Design review of the part built by this model. Coordinates are the model's own, in mm. Coordinates: 2 decimals unless noted, no trailing zeros. Order: outer loops, then holes, each group sorted by start corner. A loop starts at its lowest first (then second) coordinate and runs counter-clockwise, first axis right, second up. Notation, with made-up numbers: M -29,-38 L -22,-38 A28 ccw -22,-2 Z; hole C 82,21 d2. An arc over 180 degrees is marked long. Answer in a Markdown table with one row per item.
from build123d import *

# Parameters (mm, degrees)
SKETCH1_W                         = 25.4
SKETCH1_H                         = 25.4
BOSS_EXTRUDE1_DEPTH               = 12.7
CHAMFER1_SIZE                     = 10.16
SKETCH2_R                         = 3.175
CUT_EXTRUDE1_DEPTH                = 25.4
SKETCH3_R                         = 3.175
CUT_EXTRUDE2_DEPTH                = 10.16
F_1_4_28_TAPPED_HOLE1_D           = 5.4102
F_1_4_28_TAPPED_HOLE1_DEPTH       = 15.494
F_1_4_28_TAPPED_HOLE1_CSINK_D     = 7.62
F_1_4_28_TAPPED_HOLE1_CSINK_ANGLE = 90
F_1_4_28_TAPPED_HOLE1_TIP         = 1.625388061


with BuildPart() as part:
    # Sketch1 → Boss-Extrude1 (new body)
    with BuildSketch(Plane.XY):
        with Locations((12.7, 12.7)):
            Rectangle(SKETCH1_W, SKETCH1_H)
    extrude(amount=BOSS_EXTRUDE1_DEPTH)

    # Chamfer1
    chamfer1_edges = [part.edges().sort_by_distance(p)[0] for p in [
        (0, 0, 6.35),
    ]]
    chamfer(chamfer1_edges, length=CHAMFER1_SIZE)

    # Sketch2 → Cut-Extrude1 (cut)
    with BuildSketch(Plane(origin=(0, 25.4, 0), x_dir=(1, 0, 0), z_dir=(0, 1, 0))):
        with Locations(Location((19.05, -6.35, 0), (0, 0, 270))):
            Circle(SKETCH2_R)
    extrude(amount=-CUT_EXTRUDE1_DEPTH, mode=Mode.SUBTRACT)

    # Sketch3 → Cut-Extrude2 (cut)
    with BuildSketch(Plane(origin=(5.08, 5.08, 0), x_dir=(0, 0, 1), z_dir=(-0.7071067811865488, -0.7071067811865462, 0))):
        with Locations(Location((6.35, 0, 0), (0, 0, 270))):
            Circle(SKETCH3_R)
    extrude(amount=-CUT_EXTRUDE2_DEPTH, mode=Mode.SUBTRACT)

    # 1/4-28 Tapped Hole1
    with Locations(Plane.XY.offset(12.7)):
        with Locations((8.980256121, 8.980256121), (18.974124868, 17.78)):
            CounterSinkHole(F_1_4_28_TAPPED_HOLE1_D / 2, F_1_4_28_TAPPED_HOLE1_CSINK_D / 2, depth=F_1_4_28_TAPPED_HOLE1_DEPTH, counter_sink_angle=F_1_4_28_TAPPED_HOLE1_CSINK_ANGLE)
            with Locations((0, 0, -(F_1_4_28_TAPPED_HOLE1_DEPTH + F_1_4_28_TAPPED_HOLE1_TIP / 2))):  # 118° drill point
                Cone(0, F_1_4_28_TAPPED_HOLE1_D / 2, F_1_4_28_TAPPED_HOLE1_TIP, mode=Mode.SUBTRACT)


solid = part.part
(1) Add section A-A, the plane z = 6.35. Give the boundary of the cut face in (x, y) (3 decimals), and give its area (3 significant figures).
Return value:
| item | result |
|---|---|
| outline | M 0,10.16 L 2.835,7.325 L 10.019,14.509 L 14.509,10.019 L 7.325,2.835 L 10.16,0 L 15.875,0 L 15.875,25.4 L 0,25.4 Z; M 22.225,0 L 25.4,0 L 25.4,25.4 L 22.225,25.4 Z |
| area | 368 mm2 |
(2) Insertion check: pin 1 Ø7 at (x, y) = (8.98, 8.98) entering from -Z; pin 2 Ø3 at (x, y) = (18.97, 17.78) entering from +Z; pin 3 Ø7 at (x, y) = (8.98, 8.98) entering from +Z. Each pin has a flat end and moves straight along its axis. Give the tip position at first contact, or say it passes through.
Return value:
| item | result |
|---|---|
| pin 1 | stops at z = 0 |
| pin 2 | passes through |
| pin 3 | stops at z = 12.39 |
(3) Draft analysis for pull direction X (two halves, no side actions). For faces 1 (the flat face through (12.23, 12.3, 6.39)), 2 (the flat face through (6.28, 3.88, 3.44)), 3 (the flat face through (25.4, 13, 6)), 4 (the cylindrical face through (19.19, 12.88, 3.18)), state which applies: pulls with the +X half, pulls with the -X half, needs draft (parallel to the pull), parting line crosses it, or undercut.
Return value:
| item | result |
|---|---|
| face 1 | undercut |
| face 2 | pulls with the -X half |
| face 3 | pulls with the +X half |
| face 4 | undercut |
(4) Add section C-C, the plane z = 11.25. Give the boundary of the cut face in (x, y).
Return value:
| item | result |
|---|---|
| outline | M 0,10.16 L 10.16,0 L 25.4,0 L 25.4,25.4 L 0,25.4 Z; hole C 8.98,8.98 d5.41; hole C 18.97,17.78 d5.41 |
(5) Add section B-B, the plane y = 17.78. Give the boundary of the cut face in (x, z) (3 decimals).
Return value:
| item | result |
|---|---|
| outline | M 0,0 L 16.269,0 L 16.269,4.818 A3.175 cw 16.269,7.882 L 16.269,11.595 L 15.164,12.7 L 0,12.7 Z; M 21.679,0 L 25.4,0 L 25.4,12.7 L 22.784,12.7 L 21.679,11.595 L 21.679,8.13 A3.175 cw 21.679,4.57 Z |
(6) Add section D-D, the plane x = 19.05. Give the number of separate pieces and of enclosed holes in the cut face, and give its area (3 significant figures).
Return value:
| item | result |
|---|---|
| separate pieces | 4 |
| enclosed holes | 0 |
| area | 126 mm2 |
(7) For line 1 along X through (y, z) = (17.78, 2.8); line 2 along X through (y, z) = (16, 6.35) (3 decimals); line 3 along X through (y, z) = (9, 4.75), list the stretches that pass through material, from the lowest coordinate up. Write a range as from..to.
Return value:
| item | result |
|---|---|
| line 1 | x = 0..16.27, 21.68..25.4 |
| line 2 | x = 0..15.875, 22.225..25.4 |
| line 3 | x = 1.16..5.12, 12.88..16.31, 21.79..25.4 |
